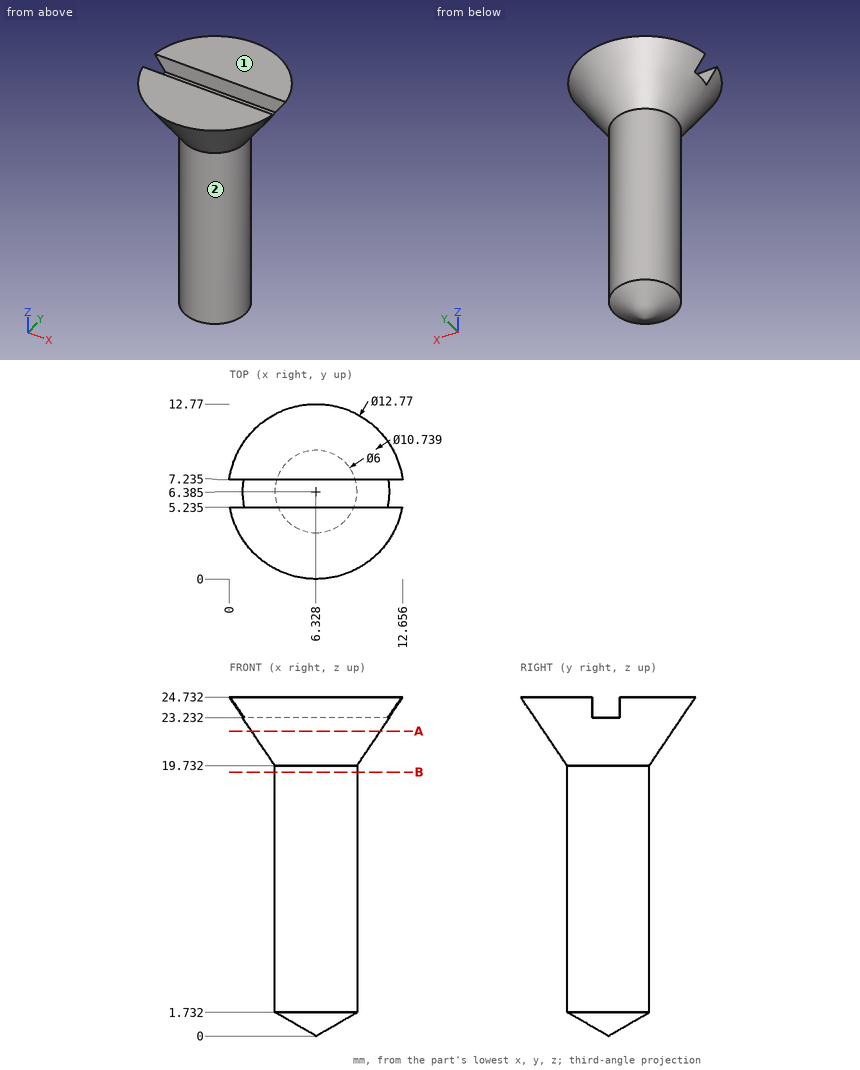
Job drawing, mm, ordinate dimensions from the low corner. One solid piece. A direction names the side the tool comes from. Round coordinates to 2 decimals unless told otherwise and drop trailing zeros. Order: outer loops, then holes, each group sorted by start corner. A loop starts at its lowest first (then second) coordinate and runs counter-clockwise, first axis right, second up. Notation, with made-up numbers: M -36,-19.75 L -16,-19.75 A29 ccw -16,1.25 Z; hole C 1,-33.5 d3. An arc over 180 degrees is marked long. Write each question's results on one line, items separated by ' | '. Start each with the question number.
(1) Saw through at A-A, the plane z = 22.25. Give the cut face in (x, y) (1 decimal).
(2) Probe probe 1 along X at (y, z) = (8, 22) (1 decimal); probe 2 along Z at (x, y) = (10, 8) (1 decimal); probe 3 along Y at (x, z) = (4.5, 2.5) (1 decimal). List the from-to ranges inside material, lowest first. Write a range as from..to.
(3) Saw through at B-B, the plane z = 19.25. Give the cut face in (x, y) (1 decimal), then the cut area to 3 significant figures.
(4) Drop flat-ended pins along their axis: pin 1 (5 mm diameter, centred on y = 4, z = 3, fed in from -X); pin 2 (3 mm diameter, centred on x = 11, z = 10, fed in from +Y); pin 3 (1.5 mm diameter, centred on x = 4, z = 19, fed in from +Y); pin 4 (3 mm diameter, centred on x = 2.5, z = 6, fed in from -Y). Give the stop position or say it passes through.
(5) Which spindle directions (+Z, -Z, +X, -X, +Y, -Y) get a long thin tool onto all of the face, cutting with end or side? Do the marked faces 1 and 2. Say none if no direction does.
Established:
1) outline: C 6.3,6.4 d9.4
2) probe 1: x = 2.1..10.6 | probe 2: z = 21.2..24.7 | probe 3: y = 4..8.8
3) outline: C 6.3,6.4 d6 | area: 28.3 mm^2
4) pin 1: stops at x = 3.33 | pin 2: passes through | pin 3: stops at y = 8.94 | pin 4: stops at y = 4.49
5) face 1: +Z, +X, -X, +Y, -Y | face 2: -Z
